Check sheet for the modelled part. Datum: model origin and axes. Units: mm. A direction names the side the tool comes from. Round coordinates to 2 decimals unless told otherwise and drop trailing zeros. Write each loop counter-clockwise with the first axis right and the second up, starting at its lowest first coordinate (ties: lowest second). Pieces come first, ordered by that corner, then holes. Notation, with made-up numbers: M 7,84 L 51,84 A26 cw 51,120 Z; hole C 29,-22 d1. An arc over 180 degrees is marked long. One line per item, written item: value.
from build123d import *

# Parameters (mm, degrees)
SKETCH1_W           = 76.32
SKETCH1_H           = 102
BOSS_EXTRUDE1_DEPTH = 6
SKETCH2_W           = 30
SKETCH2_H           = 6
BOSS_EXTRUDE2_DEPTH = 6
LPATTERN1_COUNT     = 2
LPATTERN1_PITCH     = 72
SKETCH4_W           = 30
SKETCH4_H           = 6
BOSS_EXTRUDE3_DEPTH = 6
LPATTERN2_COUNT     = 2
LPATTERN2_PITCH     = 72
SKETCH5_W           = 30
SKETCH5_H           = 6
CUT_EXTRUDE1_DEPTH  = 6


with BuildPart() as part:
    # Sketch1 → Boss-Extrude1 (new body)
    with BuildSketch(Plane(origin=(0, 0, 0), x_dir=(1, 0, 0), z_dir=(0, 1, 0))):
        with Locations((38.16, 51)):
            Rectangle(SKETCH1_W, SKETCH1_H)
    extrude(amount=BOSS_EXTRUDE1_DEPTH)

    # Sketch2 → Boss-Extrude2 (add)
    with BuildSketch(Plane(origin=(76.32, 0, 0), x_dir=(0, 0, -1), z_dir=(1, 0, 0))):
        with Locations((15, 3)):
            Rectangle(SKETCH2_W, SKETCH2_H)
    boss_extrude2 = extrude(amount=BOSS_EXTRUDE2_DEPTH)

    # LPattern1: Boss-Extrude2 ×2
    with Locations(*[(0, 0, -i * LPATTERN1_PITCH) for i in range(1, LPATTERN1_COUNT)]):
        add(boss_extrude2)

    # Sketch4 → Boss-Extrude3 (add)
    with BuildSketch(Plane.ZY):
        with Locations((-87, 3)):
            Rectangle(SKETCH4_W, SKETCH4_H)
    boss_extrude3 = extrude(amount=BOSS_EXTRUDE3_DEPTH)

    # LPattern2: Boss-Extrude3 ×2
    with Locations(*[(0, 0, i * LPATTERN2_PITCH) for i in range(1, LPATTERN2_COUNT)]):
        add(boss_extrude3)

    # Sketch5 → Cut-Extrude1 (cut)
    with BuildSketch(Plane.XY):
        with Locations((36.34, 3)):
            Rectangle(SKETCH5_W, SKETCH5_H)
    cut_extrude1 = extrude(amount=-CUT_EXTRUDE1_DEPTH, mode=Mode.SUBTRACT)

    # Mirror1: Cut-Extrude1 across plane
    add(cut_extrude1.mirror(Plane(origin=(0, 0, -51), x_dir=(1, 0, 0), z_dir=(0, 0, -1))), mode=Mode.SUBTRACT)


solid = part.part
Q1. Sectioned sample at C-C on x = 24.5. Enter the section's corners in (y, z), and give its area (3 significant figures).
Completed:
outline: M 0,-96 L 6,-96 L 6,-6 L 0,-6 Z
area: 540 mm^2
Q2. Sectioned sample at B-B on z = -41. Enter the section's corners in (x, y).
Completed:
outline: M 0,0 L 76.32,0 L 76.32,6 L 0,6 Z
Q3. Sectioned sample at A-A on y = 3.5. Enter the section's corners in (x, z), and give its area (3 significant figures).
Completed:
outline: M -6,-102 L 21.34,-102 L 21.34,-96 L 51.34,-96 L 51.34,-102 L 82.32,-102 L 82.32,-72 L 76.32,-72 L 76.32,-30 L 82.32,-30 L 82.32,0 L 51.34,0 L 51.34,-6 L 21.34,-6 L 21.34,0 L -6,0 L -6,-30 L 0,-30 L 0,-72 L -6,-72 Z
area: 8,140 mm^2
Q4. Scan lines: line 1 (X direction, y = 4.05, z = -96.5); line 2 (X direction, y = 1, z = -68); line 3 (Z direction, x = 22.5, y = 3.5). Record each from-to range of solid material in increasing order. Write a range as [from, to].
Completed:
line 1: [-6, 21.34], [51.34, 82.32]
line 2: [0, 76.32]
line 3: [-96, -6]
Q5. Depth check by flat-ended pin: P1, Ø2, axis at y = 2, z = -55.5, coming from the +X side. Enter the tip coordinate at first touch or a pass-through.
Completed:
P1: x = 76.32
Q6. Draft check along X on faces 4 (the flat face through (39, 0, -52)), 5 (the flat face through (36, 3, -96)), 6 (the flat face through (-6, 3, -15)). Enter one of: pulls with the +X half, pulls with the -X half, needs draft (parallel to the pull), parting line crosses it, or undercut.
Completed:
face 4: needs draft
face 5: undercut
face 6: pulls with the -X half
Q7. Access from +Z, -Z, +X, -X, +Y, -Y to the whole of each face (thin tool, end or side, straight path). Record for faces 1 (the flat face through (51.34, 3, -3)), 2 (the flat face through (-3, 3, -30)), 3 (the flat face through (51.34, 3, -99)).
Completed:
face 1: +Z, +Y, -Y
face 2: -X, +Y, -Y
face 3: -Z, +Y, -Y
